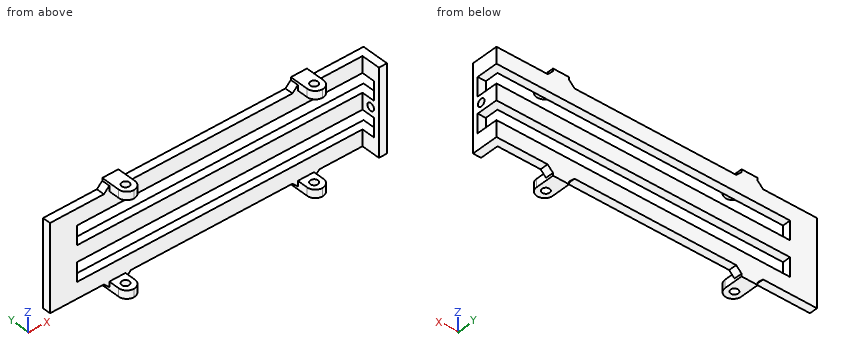
from build123d import *

# Parameters (mm, degrees)
SKETCH1_W           = 119
SKETCH1_H           = 32
SKETCH1_W_2         = 105
SKETCH1_H_2         = 7
BOSS_EXTRUDE1_DEPTH = 3
SKETCH2_W           = 6
SKETCH2_H           = 7
SKETCH2_R           = 1.4
SKETCH2_H_2         = 3
BOSS_EXTRUDE2_DEPTH = 3
CHAMFER1_SIZE       = 2
FILLET1_R           = 3
SKETCH3_W           = 3
SKETCH3_H           = 11
BOSS_EXTRUDE4_DEPTH = 32
SKETCH4_W           = 4
SKETCH4_H           = 7
CUT_EXTRUDE1_DEPTH  = 8
SKETCH5_R           = 1.4
CUT_EXTRUDE2_DEPTH  = 122.008264181
SKETCH6_W           = 32
SKETCH6_H           = 4
CUT_EXTRUDE3_DEPTH  = 10


with BuildPart() as part:
    # Sketch1 → Boss-Extrude1 (new body)
    with BuildSketch(Plane(origin=(0, 0, 0), x_dir=(1, 0, 0), z_dir=(0, 1, 0))):
        Rectangle(SKETCH1_W, SKETCH1_H)
        with Locations((3, 6.5)):
            Rectangle(SKETCH1_W_2, SKETCH1_H_2, mode=Mode.SUBTRACT)
        with Locations((3, -6.5)):
            Rectangle(SKETCH1_W_2, SKETCH1_H_2, mode=Mode.SUBTRACT)
    extrude(amount=BOSS_EXTRUDE1_DEPTH)

    # Sketch2 → Boss-Extrude2 (add)
    # profile 1 of 4: a face of its own
    with BuildSketch(Plane.XY.offset(16)):
        with Locations((35.5, -3.5)):
            Rectangle(SKETCH2_W, SKETCH2_H)
        with Locations((35.5, -3.5)):
            Circle(SKETCH2_R, mode=Mode.SUBTRACT)
    # profile 2 of 4: a face of its own
    with BuildSketch(Plane.XY.offset(16)):
        with Locations((35.5, 1.5)):
            Rectangle(SKETCH2_W, SKETCH2_H_2)
    # profile 3 of 4: a face of its own
    with BuildSketch(Plane.XY.offset(16)):
        with Locations((-34.5, -3.5)):
            Rectangle(SKETCH2_W, SKETCH2_H)
        with Locations((-34.5, -3.5)):
            Circle(SKETCH2_R, mode=Mode.SUBTRACT)
    # profile 4 of 4: a face of its own
    with BuildSketch(Plane.XY.offset(16)):
        with Locations((-34.5, 1.5)):
            Rectangle(SKETCH2_W, SKETCH2_H_2)
    boss_extrude2 = extrude(amount=BOSS_EXTRUDE2_DEPTH)

    # Mirror4: Boss-Extrude2 across plane
    add(boss_extrude2.mirror(Plane.XY))

    # Chamfer1
    chamfer1_edges = [part.edges().sort_by_distance(p)[0] for p in [
        (-31.5, 1.5, -16),
        (38.5, 1.5, 16),
        (32.5, 1.5, 16),
        (-37.5, 1.5, 16),
        (-31.5, 1.5, 16),
        (32.5, 1.5, -16),
        (38.5, 1.5, -16),
        (-37.5, 1.5, -16),
    ]]
    chamfer(chamfer1_edges, length=CHAMFER1_SIZE)

    # Fillet1
    fillet1_edges = [part.edges().sort_by_distance(p)[0] for p in [
        (32.5, -7, 17.5),
        (38.5, -7, 17.5),
        (-37.5, -7, 17.5),
        (-31.5, -7, 17.5),
        (38.5, -7, -17.5),
        (32.5, -7, -17.5),
        (-31.5, -7, -17.5),
        (-37.5, -7, -17.5),
    ]]
    fillet(fillet1_edges, radius=FILLET1_R - 0.0001)  # a hair under: the kernel refuses the full size

    # Sketch3 → Boss-Extrude4 (add)
    with BuildSketch(Plane(origin=(0, 0, -16), x_dir=(-1, 0, 0), z_dir=(0, 0, -1))):
        with Locations((-58, -5.5)):
            Rectangle(SKETCH3_W, SKETCH3_H)
    extrude(amount=-BOSS_EXTRUDE4_DEPTH)

    # Sketch4 → Cut-Extrude1 (cut)
    with BuildSketch(Plane(origin=(0, 3, 0), x_dir=(1, 0, 0), z_dir=(0, 1, 0))):
        with Locations((57.5, 6.5)):
            Rectangle(SKETCH4_W, SKETCH4_H)
        with Locations((57.5, -6.5)):
            Rectangle(SKETCH4_W, SKETCH4_H)
    extrude(amount=-CUT_EXTRUDE1_DEPTH, mode=Mode.SUBTRACT)

    # Sketch5 → Cut-Extrude2 (cut, through all)
    with BuildSketch(Plane(origin=(59.5, 0, 0), x_dir=(0, 0, -1), z_dir=(1, 0, 0))):
        with Locations((0, -3.5)):
            Circle(SKETCH5_R)
    extrude(amount=-CUT_EXTRUDE2_DEPTH, mode=Mode.SUBTRACT)

    # Sketch6 → Cut-Extrude3 (cut)
    with BuildSketch(Plane(origin=(59.5, 0, 0), x_dir=(0, 0, -1), z_dir=(1, 0, 0))):
        with Locations((0, -9)):
            Rectangle(SKETCH6_W, SKETCH6_H)
    extrude(amount=-CUT_EXTRUDE3_DEPTH, mode=Mode.SUBTRACT)


solid = part.part
The listing builds one solid part. Answer for the finished solid, in the listing's coordinates (mm). Give positions to 0.01 mm unless a question says otherwise; leave off trailing zeros. Order: outer loops, then holes, each group sorted by start corner. A loop starts at its lowest first (then second) coordinate and runs counter-clockwise, first axis right, second up. Notation, with made-up numbers: (70, 35.25) -> (97, 35.25) arc R30 cw to (97, 61.25) -> close; hole circle Ø11 at (15.5, -23.75). An arc over 180 degrees is marked (long way). Put each result on its own line as item: value.
Item 1: A cutting plane is placed at D-D on z = 14.5. Give the vertices of the cut face in (x, y), plus the area to 3 significant figures.
Established:
outline: (-59.5, 0) -> (56.5, 0) -> (56.5, -7) -> (59.5, -7) -> (59.5, 3) -> (-59.5, 3) -> close
area: 378 mm^2
Item 2: A cutting plane is placed at B-B on x = -0.5. Give the vertices of the cut face in (y, z).
Established:
outline: (0, -16) -> (3, -16) -> (3, -10) -> (0, -10) -> close; (0, -3) -> (3, -3) -> (3, 3) -> (0, 3) -> close; (0, 10) -> (3, 10) -> (3, 16) -> (0, 16) -> close
Item 3: Straight lines are drawn through the part: line 1 (Z direction, x = 50, y = 1.25); line 2 (Y direction, x = 57, z = 0); line 3 (X direction, y = -5.5, z = -10.5). For each, find the intervals that lie inside material, in ascending order.
Established:
line 1: z = -16 to -10, -3 to 3, 10 to 16
line 2: y = -7 to -4.9, -2.1 to 3
line 3: x = 56.5 to 59.5
Item 4: A cutting plane is placed at A-A on z = -5.5. Give the vertices of the cut face in (x, y).
Established:
outline: (-59.5, 0) -> (-49.5, 0) -> (-49.5, 3) -> (-59.5, 3) -> close; (56.5, -7) -> (59.5, -7) -> (59.5, -5) -> (56.5, -5) -> close
Item 5: A cutting plane is placed at C-C on z = 0. Give the vertices of the cut face in (x, y).
Established:
outline: (-59.5, 0) -> (56.5, 0) -> (56.5, -2.1) -> (59.5, -2.1) -> (59.5, 3) -> (-59.5, 3) -> close; (56.5, -7) -> (59.5, -7) -> (59.5, -4.9) -> (56.5, -4.9) -> close
Item 6: Given P1, Ø5, axis at x = -7.5, z = -2, coming from the -Y side; P2, Ø3.5, axis at x = -1, y = 1.5, coming from the +Z side; P3, Ø2.5, axis at y = -0.5, z = 17.5, coming from the +X side, each flat-ended and moving along its own axis, determine where each tip first touches the part or whether it passes through.
Established:
P1: stops at y = 0
P2: stops at z = 16
P3: stops at x = 40.15
